Autodesk Inventor part; units mm, degrees
ref_plane "Work Plane1" through (0, 0, 11) normal (1, 0, 0) x (0, 0, -1)
ref_plane "YZ Plane" through (0, 0, 0) normal (1, 0, 0) x (0, 1, 0)
ref_plane "XZ Plane" through (0, 0, 0) normal (0, 1, 0) x (-1, 0, 0)
sketch "Эскиз1" plane through (0, 0, 0) normal (0, 1, 0) x (-1, 0, 0)
  line L0 (5.5, 11.5) -> (-5.5, 11.5)
  line L1 (-6, 11) -> (-6, -11)
  line L2 (-5.5, -11.5) -> (5.5, -11.5)
  line L3 (6, -11) -> (6, 11)
  line L4 (6, 11.5) -> (-6, -11.5) construction
  line L5 (-6, 11.5) -> (6, -11.5) construction
  arc A0 (6, 11) -> (5.5, 11.5) centre (5.5, 11) ccw
  arc A1 (5.5, -11.5) -> (6, -11) centre (5.5, -11) ccw
  arc A2 (-6, -11) -> (-5.5, -11.5) centre (-5.5, -11) ccw
  arc A3 (-5.5, 11.5) -> (-6, 11) centre (-5.5, 11) ccw
  point P0 (0, 0)
  dimension "d0" = 12
  dimension "d1" = 23
  dimension "d2" = 0.5
extrude "Выдавливание1" add sketch "Эскиз1" along normal blind 16
sketch "Эскиз2" plane through (0, 16, 0) normal (0, 1, 0) x (1, 0, 0)
  line L0 (6, -16.25) -> (6, 16.25)
  line L1 (-6, 16.25) -> (-6, -16.25)
  line L2 (-6, -16.25) -> (6, 16.25) construction
  line L3 (6, -16.25) -> (-6, 16.25) construction
  arc A0 (0.5, -14.366) -> (-0.5, -14.366) centre (0, -13.5) ccw
  arc A1 (-0.5, 14.366) -> (0.5, 14.366) centre (0, 13.5) ccw
  line L4 (-0.5, -14.366) -> (-0.5, -16.25)
  line L5 (0.5, -14.366) -> (0.5, -16.25)
  line L6 (-6, -16.25) -> (-0.5, -16.25)
  line L7 (0.5, -16.25) -> (6, -16.25)
  line L8 (-0.5, 14.366) -> (-0.5, 16.25)
  line L9 (0.5, 14.366) -> (0.5, 16.25)
  line L10 (6, 16.25) -> (0.5, 16.25)
  line L11 (-0.5, 16.25) -> (-6, 16.25)
  point P0 (0, 0)
  point P1 (0, 0)
  point P2 (0, 0)
  dimension "d5" = 12
  dimension "d6" = 32.5
  dimension "d7" = 2
  dimension "d8" = 2
  dimension "d9" = 1
  dimension "d10" = 0.5
  dimension "d13" = 27
  dimension "d14" = 13.5
extrude "Выдавливание2" add sketch "Эскиз2" along normal blind 2
sketch "Эскиз3" plane through (0, 18, 0) normal (0, 1, 0) x (1, 0, 0)
  line L0 (6, -16.25) -> (6, 16.25)
  line L1 (-6, -11.25) -> (6, -11.25)
  line L2 (6, -11.25) -> (6, 11.25)
  line L3 (6, 11.25) -> (-6, 11.25)
  line L4 (-6, 11.25) -> (-6, -11.25)
  line L5 (-6, -11.25) -> (6, 11.25) construction
  line L6 (6, -11.25) -> (-6, 11.25) construction
  point P0 (0, 0)
  dimension "d15" = 22.5
  dimension "d18" = 12
extrude "Выдавливание3" add sketch "Эскиз3" along normal blind 5
sketch "Эскиз4" plane through (0, 23, 0) normal (0, 1, 0) x (1, 0, 0)
  arc A0 (-2.75, -0.2002) -> (2.75, -0.2002) centre (0, -5.25) ccw
  arc A1 (2.75, 0.75) -> (-2.75, 0.75) centre (0, 0.75) ccw
  line L0 (-2.75, 0.75) -> (-2.75, -0.2002)
  line L1 (2.75, 0.75) -> (2.75, -0.2002)
  line L2 (-6, -11.25) -> (6, -11.25)
  point P0 (0, 0)
  dimension "d19" = 11.5
  dimension "d20" = 5.25
  dimension "d21" = 5.5
  dimension "d22" = 6
  dimension "d23" = 11.25
extrude "Выдавливание4" add sketch "Эскиз4" along normal blind 4
fillet "Сопряжение1" radius 0.25 4 edges at (0, 27, 11) (0, 27, -3.5) (2.75, 27, -0.2749) (-2.75, 27, -0.2749)
sketch "Эскиз5" plane through (0, 23, 0) normal (0, 1, 0) x (1, 0, 0)
  line L0 (-4.25, 4.75) -> (4.25, 4.75)
  line L1 (4.5, 5) -> (4.5, 9.5)
  line L2 (4.25, 9.75) -> (-4.25, 9.75)
  line L3 (-4.5, 9.5) -> (-4.5, 5)
  line L4 (6, 11.25) -> (-6, 11.25)
  line L5 (-6, 11.25) -> (-6, -11.25)
  line L6 (6, -11.25) -> (6, 11.25)
  arc A0 (-4.5, 5) -> (-4.25, 4.75) centre (-4.25, 5) ccw
  arc A1 (-4.25, 9.75) -> (-4.5, 9.5) centre (-4.25, 9.5) ccw
  arc A2 (4.5, 9.5) -> (4.25, 9.75) centre (4.25, 9.5) ccw
  arc A3 (4.25, 4.75) -> (4.5, 5) centre (4.25, 5) ccw
  point P0 (0, 0)
  dimension "d27" = 1.5
  dimension "d28" = 1.5
  dimension "d29" = 1.5
  dimension "d30" = 5
  dimension "d31" = 0.25
extrude "Выдавливание5" cut sketch "Эскиз5" against normal blind 0.25
sketch "Эскиз6" plane through (0, 27, 0) normal (0, 1, 0) x (1, 0, 0)
  arc A0 (-2.5, -0.351) -> (2.5, -0.351) centre (0, -5.25) ccw
  circle A1 centre (0, -5.25) radius 2.25
  circle A2 centre (0, -5.25) radius 0.5
  point P0 (0, 0)
  dimension "d34" = 4.5
  dimension "d35" = 1
extrude "Выдавливание6" add sketch "Эскиз6" along normal blind 3
ref_plane "Work Plane1" through (0, 0, 11) normal (1, 0, 0) x (0, 0, -1)
equation "\"d8\" = d7"
equation "\"d28\" = d27"
equation "\"d29\" = d27"
equation "\"d45\" = 0.5 * d44"
properties part number "Servomotor HTX900" material "Поликарбонат, дымчатый"
The model under review builds one solid part; all positions refer to its coordinate system, in mm. A direction names the side the tool comes from. Round coordinates to 2 decimals unless told otherwise and drop trailing zeros. Loops run counter-clockwise (first coordinate to the right, second up) from the corner with the lowest first, then second, coordinate; pieces in that order, holes last. Notation, with made-up numbers: M 7.25,51.5 L 21.25,51.5 A21 ccw 21.25,83.5 Z; hole C 34,36.25 d9. An arc over 180 degrees is marked long. Answer as a JSON object with one key per item and string values.
Item 1: We need section B-B, the plane z = 5.25. State the section outline as (x, y) points.
Check sheet entries:
{"outline": "M -6,0 L 6,0 L 6,23 L 5.75,23 L 5.75,26.75 A0.25 ccw 5.5,27 L 2.25,27 L 2.25,30 L 0.5,30 L 0.5,27 L -0.5,27 L -0.5,30 L -2.25,30 L -2.25,27 L -5.5,27 A0.25 ccw -5.75,26.75 L -5.75,23 L -6,23 Z"}
Item 2: The part is to be moulded in two halves that separate along X. For faces 6 (the face through (-2.75, 25, 0)), 7 (the face through (0, 25, 11)), 8 (the face through (0, 22.75, -7)), 9 (the face through (1.2, 18, -13.8)), say which applies: +X half, -X half, draft (parallel to the pull), parting line (faces both ways), or undercut.
Check sheet entries:
{"face 6": "-X half", "face 7": "parting line", "face 8": "undercut", "face 9": "draft"}
Item 3: We need section C-C, the plane y = 9.5. State the section outline as (x, z) points, and give its area (3 significant figures).
Check sheet entries:
{"outline": "M -6,-11 A0.5 ccw -5.5,-11.5 L 5.5,-11.5 A0.5 ccw 6,-11 L 6,11 A0.5 ccw 5.5,11.5 L -5.5,11.5 A0.5 ccw -6,11 Z", "area": "276 mm2"}
Item 4: For line 1 along X through (y, z) = (28.5, 5.25); line 2 along Z through (x, y) = (0, 29.1); line 3 along X through (y, z) = (17.4, 13.5), list the stretches that pass through material, from the lowest coordinate up.
Check sheet entries:
{"line 1": "-2.25 to -0.5, 0.5 to 2.25", "line 2": "3 to 4.75, 5.75 to 7.5", "line 3": "-6 to -1, 1 to 6"}
Item 5: Tool access review of faces 1 (the face through (0, 20, 11.25)), 2 (the face through (-0.5, 17, 15)), 3 (the face through (0, 20, -11.25)), 4 (the face through (0, 27, 5)), 5 (the face through (0, 8, -11.5)): name each direction out of +Z, -Z, +X, -X, +Y, -Y from which nothing blocks a thin tool from reaching the whole face with its end or side.
Check sheet entries:
{"face 1": "+Z, +X, -X, +Y", "face 2": "+Z, +Y, -Y", "face 3": "-Z, +X, -X, +Y", "face 4": "+Y", "face 5": "-Z, +X, -X, -Y"}
Item 6: Clearance check with flat-ended pins moving along their axes: P1, Ø5.5, axis at x = 2.5, y = 11.5, coming from the -Z side; P2, Ø2.5, axis at x = 0, z = 13.5, coming from the -Y side; P3, Ø3.5, axis at x = 1.5, y = 6.5, coming from the +Z side; P4, Ø1.2, axis at x = 0, z = -13.5, coming from the +Y side. State where each tip first meets the part, or that it passes through.
Check sheet entries:
{"P1": "z = -11.5", "P2": "y = 16", "P3": "z = 11.5", "P4": "through"}
Item 7: We need section A-A, the plane z = -13.5. State the section outline as (x, y) points.
Check sheet entries:
{"outline": "M -6,16 L -1,16 L -1,18 L -6,18 Z; M 1,16 L 6,16 L 6,18 L 1,18 Z"}
